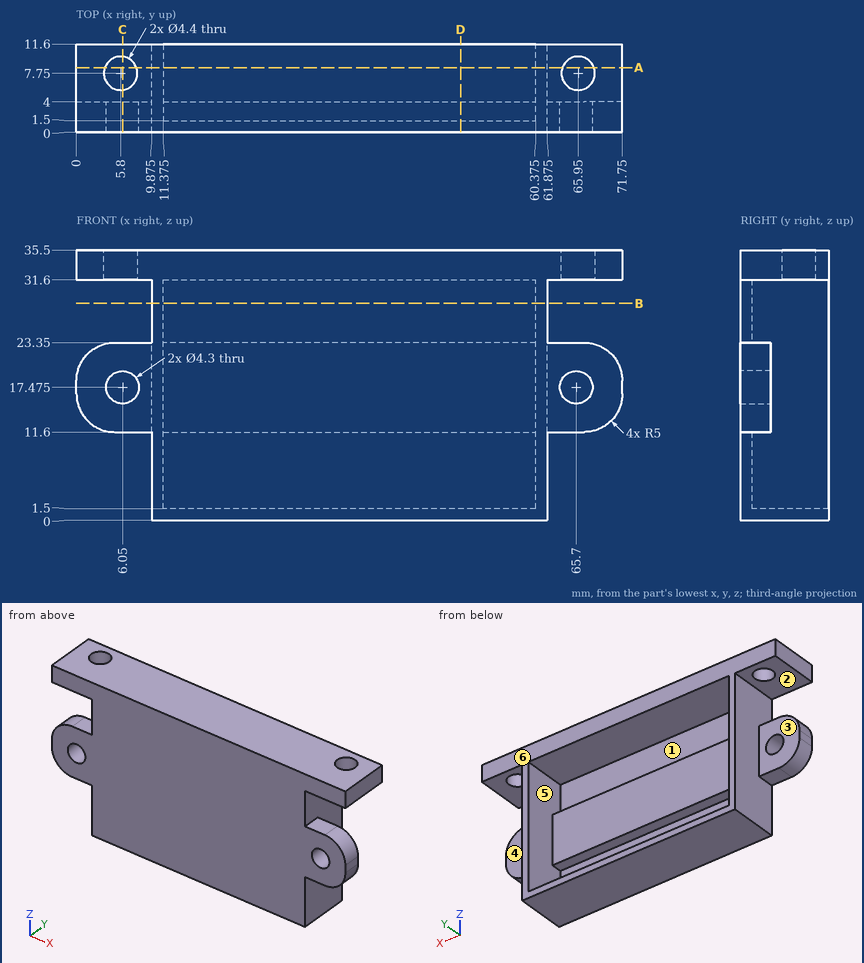
The figure shows three views and two pictorial views of one solid part (mm, origin at its lowest corner). Answer the questions. A direction names the side the tool comes from. Give positions to 0.01 mm unless a question says otherwise; leave off trailing zeros. Write each loop counter-clockwise with the first axis right and the second up, starting at its lowest first coordinate (ties: lowest second). Pieces come first, ordered by that corner, then holes. Notation, with made-up numbers: (25, -17.5) -> (58, -17.5) arc R10 ccw to (58, -5.5) -> close; hole circle Ø9 at (-6.5, -24). An arc over 180 degrees is marked (long way). Answer as a JSON object with one key per item and string values.
1) Section D-D on x = 50.5 is taken. Write down the section's boundary in (y, z), then the cut area to 3 significant figures.
Findings below:
{"outline": "(0, 0) -> (11.6, 0) -> (11.6, 1.5) -> (1.5, 1.5) -> (1.5, 11.6) -> (4, 11.6) -> (4, 23.35) -> (1.5, 23.35) -> (1.5, 31.6) -> (11.6, 31.6) -> (11.6, 35.5) -> (0, 35.5) -> close", "area": "137 mm^2"}
2) Section A-A on y = 8.5 is taken. Write down the section's boundary in (x, z) (3 decimals).
Findings below:
{"outline": "(0, 31.6) -> (3.732, 31.6) -> (3.732, 35.5) -> (0, 35.5) -> close; (7.868, 31.6) -> (9.875, 31.6) -> (9.875, 0) -> (61.875, 0) -> (61.875, 31.6) -> (63.882, 31.6) -> (63.882, 35.5) -> (7.868, 35.5) -> close; (68.018, 31.6) -> (71.75, 31.6) -> (71.75, 35.5) -> (68.018, 35.5) -> close; hole (11.375, 1.5) -> (60.375, 1.5) -> (60.375, 31.6) -> (11.375, 31.6) -> close"}
3) For a pull along X with two mould halves and no side action, classify the marked faces 5 and 6 as pulls with the +X half, pulls with the -X half, needs draft (parallel to the pull), parting line crosses it, or undercut.
Findings below:
{"face 5": "undercut", "face 6": "needs draft"}
4) Section B-B on z = 28.5 is taken. Write down the section's boundary in (x, y) (3 decimals), then the cut area to 3 significant figures.
Findings below:
{"outline": "(9.875, 0) -> (61.875, 0) -> (61.875, 11.6) -> (60.375, 11.6) -> (60.375, 1.5) -> (11.375, 1.5) -> (11.375, 11.6) -> (9.875, 11.6) -> close", "area": "108 mm^2"}
5) A tool of negligible diameter and unlimited length cuts with its end or side. For the marked faces 1, 2, 3 and 4, from which of +Z, -Z, +X, -X, +Y, -Y can it reach the whole face along a straight path? Write none if from no direction.
Findings below:
{"face 1": "+Y", "face 2": "-X, +Y, -Y", "face 3": "-Z, -X, +Y", "face 4": "-Z, +X, +Y"}
6) Straight lines are drawn through the part: probe 1 along Z at (x, y) = (42.5, 2.75); probe 2 along Z at (x, y) = (54, 7.75); probe 3 along X at (y, z) = (1.75, 8) (3 decimals). For each, find the intervals that lie inside material, in ascending order. Write a range as from..to.
Findings below:
{"probe 1": "z = 0..1.5, 11.6..23.35, 31.6..35.5", "probe 2": "z = 0..1.5, 31.6..35.5", "probe 3": "x = 9.875..11.375, 60.375..61.875"}
7) Flat-ended cylindrical pins translate along their axes: pin 1 Ø5 at (x, z) = (7, 18) entering from +Y; pin 2 Ø5 at (x, z) = (41.5, 4.5) entering from +Y; pin 3 Ø2 at (x, y) = (8, 2.5) entering from -Z. Find the tip coordinate at first contact, or state that the pin passes through.
Findings below:
{"pin 1": "stops at y = 4", "pin 2": "stops at y = 1.5", "pin 3": "stops at z = 11.6"}
8) Section C-C on x = 6.05 is taken. Write down the section's boundary in (y, z) (3 decimals), then the cut area to 3 significant figures.
Findings below:
{"outline": "(0, 11.6) -> (4, 11.6) -> (4, 15.325) -> (0, 15.325) -> close; (0, 19.625) -> (4, 19.625) -> (4, 23.35) -> (0, 23.35) -> close; (0, 31.6) -> (5.564, 31.6) -> (5.564, 35.5) -> (0, 35.5) -> close; (9.936, 31.6) -> (11.6, 31.6) -> (11.6, 35.5) -> (9.936, 35.5) -> close", "area": "58.0 mm^2"}
